Build history of the part. All positions in model axes, mm. A direction names the side the tool comes from. Give positions to 0.01 mm unless a question says otherwise; leave off trailing zeros. Write item = value, one per line. Start each with the question number.
Q1. Drop flat-ended pins along their axis: P1, Ø2, axis at x = 4.5, y = 7.5, coming from the -Z side; P2, Ø4, axis at x = -0.5, z = 6, coming from the -Y side; P3, Ø1.8, axis at x = -7, y = 10, coming from the -Z side; P4, Ø3, axis at x = -11, z = 25, coming from the +Y side. Give the stop position or say it passes through.
Q2. Wall check: line 1 (Y direction, x = -0.25, z = 26.5); line 2 (X direction, y = 3, z = 3.5); line 3 (Y direction, x = 0, z = 10.25). Give the ranges that are in metal, low to high.
Q3. Tool access for faces 5 (the face through (6.466, -2.681, 12.675)), 6 (the face through (6.259, -4.232, 35.233)): list every direction of +Z, -Z, +X, -X, +Y, -Y with a clear straight run to the whole face (end or side of a thin tool).
Q4. Saw through at A-A, the plane x = -5.25. Give the number of separate pieces and of enclosed holes in the cut face, then the cut area to 3 significant figures.
Q5. Mould opens along Y. For faces 1 (the face through (4, 0, 35)), 2 (the face through (-9.105, 8.733, 31.76)), 3 (the face through (7.5, 10.4, 30)), 4 (the face through (-3.01, -12.25, 31.76)) say: pulls with the +Y half, pulls with the -Y half, needs draft (parallel to the pull), parting line crosses it, or undercut.
from build123d import *

# Parameters (mm, degrees)
F2_R      = 4.75
F3_DEPTH  = 5
F5_DEPTH  = 1.5
F6_R      = 2
F7_DEPTH  = 30
F8_R      = 2
F9_DEPTH  = 30
F10_R     = 2
F11_DEPTH = 30


with BuildPart() as f1:
    # F0 (on Front) → F1 (revolve)
    with BuildSketch(Plane.XZ):
        with BuildLine():
            Line((9.5, 25), (9.5, 3))
            ThreePointArc((9.5, 3), (10.37868, 0.87868), (12.5, 0))
            Line((12.5, 0), (12.5, 25))
            Line((12.5, 25), (12.5, 30))
            Line((12.5, 30), (4.672674, 30))
            Line((4.672674, 30), (4.672674, 25))
            Line((4.672674, 25), (7, 0))
            Line((7, 0), (7, 25))
            Line((7, 25), (9.5, 25))
        make_face()
    revolve(axis=Axis((0, 0, 27.631196), (0, 0, 1)))

    # F2 (on face) → F3 (join)
    with BuildSketch(Plane.XY.offset(30)):
        Polygon((-8.491879, -11.671389), (5.86178, -13.189877), (14.353659, -1.518488), (8.491879, 11.671389), (-5.86178, 13.189877), (-14.353659, 1.518488), align=None)
        Circle(F2_R, mode=Mode.SUBTRACT)
    extrude(amount=F3_DEPTH)

    # F4 (on face) → F5 (join)
    with BuildSketch(Plane.XY.offset(35)):
        Polygon((-5.86178, 13.189877), (-14.353659, 1.518488), (-8.491879, -11.671389), (5.86178, -13.189877), (14.353659, -1.518488), (8.491879, 11.671389), align=None)
    extrude(amount=F5_DEPTH)

    # F6 (on face) → F7 (cut)
    with BuildSketch(Plane(origin=(-1.315049, -12.430633, 0), x_dir=(0.994451, -0.105204, 0), z_dir=(-0.105204, -0.994451, 0))):
        with Locations((0, 33.25)):
            Circle(F6_R)
    extrude(amount=-F7_DEPTH, mode=Mode.SUBTRACT)

    # F8 (on face) → F9 (cut)
    with BuildSketch(Plane(origin=(-10.10772, 7.354183, 0), x_dir=(-0.588335, -0.808618, 0), z_dir=(-0.808618, 0.588335, 0))):
        with Locations((0, 33.25)):
            Circle(F8_R)
    extrude(amount=-F9_DEPTH, mode=Mode.SUBTRACT)

    # F10 (on face) → F11 (cut)
    with BuildSketch(Plane(origin=(11.422769, 5.076451, 0), x_dir=(-0.406116, 0.913822, 0), z_dir=(0.913822, 0.406116, 0))):
        with Locations((0, 33.25)):
            Circle(F10_R)
    extrude(amount=-F11_DEPTH, mode=Mode.SUBTRACT)


solid = f1.part
Report:
q1.P1 = 1.81
q1.P2 = -12.5
q1.P3 = 0
q1.P4 = 8.12
q2.line_1 = -12.5 to -4.67, 4.67 to 12.5
q2.line_2 = -12.13 to -9.01, -6.32 to -5.96, 5.96 to 6.32, 9.01 to 12.13
q2.line_3 = -12.5 to -9.5, -7 to -6.05, 6.05 to 7, 9.5 to 12.5
q3.face_5 = -Z
q3.face_6 = none
q4.separate_pieces = 1
q4.enclosed_holes = 2
q4.area = 533 mm2
q5.face_1 = undercut
q5.face_2 = pulls with the +Y half
q5.face_3 = needs draft
q5.face_4 = pulls with the -Y half
